Can you work these out from the model? Positions are in its coordinate system, mm. Face numbers are marked on the shaded views. A direction names the side the tool comes from. Round coordinates to 2 decimals unless told otherwise and drop trailing zeros. Write each loop counter-clockwise with the first axis right and the second up, starting at its lowest first coordinate (ties: lowest second). Pieces come first, ordered by that corner, then holes. Notation, with made-up numbers: (38, 29) - (96, 29) arc R9 cw to (96, 38) - close; hole circle Ø1 at (61, 77). An arc over 180 degrees is marked (long way). One line per item, written item: value. Start each with the question number.
(1) I want a section at C-C on z = 23. List the corners of the cut face in (x, y) for me.
(2) If I drill on L1, parallel to X at y = 10, z = 32; L2, parallel to X at y = 15.5, z = 24, over which ranges is the centre line in solid material (lowest first)? Write a range as from..to.
(3) I want a section at A-A on y = 18. List the corners of the cut face in (x, z) for me.
(4) On a 3-axis mill with a long thin cutter (end or side, diameter ignored), from which of +Z, -Z, +X, -X, +Y, -Y can I reach the whole of each face in a straight line? I mean the marked faces 1 and 2. Say none if no direction works.
(5) I want a section at B-B on x = 11.5. List the corners of the cut face in (y, z) for me, plus the area to 3 significant figures.
(6) I'm going to push flat-ended pins straight in: pin 1 Ø12 at (y, z) = (5.5, 18.5) entering from +X; pin 2 Ø2 at (x, z) = (33.5, 23.5) entering from -Y; pin 3 Ø16 at (x, y) = (30.5, 11) entering from +Z. Where does each tip first touch, or does it pass through?
(7) I want a section at D-D on y = 12. List the corners of the cut face in (x, z) for me, plus the area to 3 significant figures.
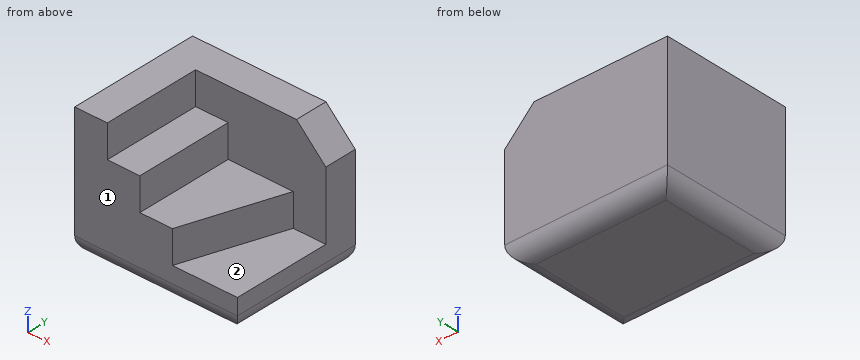
from build123d import *

# Parameters (mm, degrees)
F1_DEPTH = 40
F0_W     = 10
F0_H     = 30
F2_DEPTH = 30
F3_DEPTH = 20
F4_DEPTH = 10
F5_SIZE  = 9
F6_R     = 5


with BuildPart() as f1:
    # F0 (on Top) → F1 (new body)
    with BuildSketch(Plane.XY):
        Polygon((0, 40), (0, 0), (10, 0), (10, 30), (20, 30), (40, 30), (50, 30), (50, 40), align=None)
    extrude(amount=F1_DEPTH)

    # F0 (on Top) → F2 (join)
    with BuildSketch(Plane.XY):
        with Locations((15, 15)):
            Rectangle(F0_W, F0_H)
    extrude(amount=F2_DEPTH)

    # F0 (on Top) → F3 (join)
    with BuildSketch(Plane.XY):
        Polygon((20, 30), (20, 0), (30, 0), (40, 30), align=None)
    extrude(amount=F3_DEPTH)

    # F0 (on Top) → F4 (join)
    with BuildSketch(Plane.XY):
        Polygon((40, 30), (30, 0), (50, 0), (50, 30), align=None)
    extrude(amount=F4_DEPTH)

    # F5
    f5_edges = [f1.edges().sort_by_distance(p)[0] for p in [
        (50, 35, 40),
    ]]
    chamfer(f5_edges, length=F5_SIZE)

    # F6
    f6_edges = [f1.edges().sort_by_distance(p)[0] for p in [
        (50, 20, 0),
        (25, 0, 0),
        (0, 20, 0),
        (25, 40, 0),
    ]]
    fillet(f6_edges, radius=F6_R)


solid = f1.part
Established:
1. outline: (0, 0) - (20, 0) - (20, 30) - (50, 30) - (50, 40) - (0, 40) - close
2. L1: 0..10
2. L2: 0..20
3. outline: (0, 5) arc R5 ccw to (5, 0) - (45, 0) arc R5 ccw to (50, 5) - (50, 10) - (36, 10) - (36, 20) - (20, 20) - (20, 30) - (10, 30) - (10, 40) - (0, 40) - close
4. face 1: +Z, -Z, +X, -X, -Y
4. face 2: +Z, +X, -Y
5. outline: (0, 5) arc R5 ccw to (5, 0) - (35, 0) arc R5 ccw to (40, 5) - (40, 40) - (30, 40) - (30, 30) - (0, 30) - close
5. area: 1,290 mm2
6. pin 1: x = 33.83
6. pin 2: y = 30
6. pin 3: z = 20
7. outline: (0, 5) arc R5 ccw to (5, 0) - (45, 0) arc R5 ccw to (50, 5) - (50, 10) - (34, 10) - (34, 20) - (20, 20) - (20, 30) - (10, 30) - (10, 40) - (0, 40) - close
7. area: 1,130 mm2
